Can you work these out from the model? Positions are in its coordinate system, mm. A direction names the side the tool comes from. Give positions to 0.01 mm unless a question says otherwise; leave off trailing zeros. Order: outer loops, then holes, each group sorted by start corner. A loop starts at its lowest first (then second) coordinate and runs counter-clockwise, first axis right, second up. Notation, with made-up numbers: M -17.75,31.25 L 35.25,31.25 A10 ccw 35.25,49.25 Z; hole C 16.5,10 d9. An arc over 180 degrees is marked long. Answer as a JSON object with one key per item and string values.
```python
from build123d import *

# Parameters (mm, degrees)
SKETCH_1_W          = 10
SKETCH_1_H          = 19
EXTRUDE_1_DEPTH     = 10
SKETCH_3_R          = 2.1
CUT_EXTRUDE_2_DEPTH = 15.671400751
CUT_EXTRUDE_4_DEPTH = 5
SKETCH_2_R          = 1.5
CUT_EXTRUDE_1_DEPTH = 10


with BuildPart() as part:
    # 草图1 → 凸台-拉伸1 (new body)
    with BuildSketch(Plane.XY):
        Rectangle(SKETCH_1_W, SKETCH_1_H)
    extrude(amount=EXTRUDE_1_DEPTH)

    # 草图3 → 切除-拉伸2 (cut, through all)
    with BuildSketch(Plane(origin=(0, 0, 0), x_dir=(-1, 0, 0), z_dir=(0, 0, -1))):
        with Locations((0, 6)):
            Circle(SKETCH_3_R)
    extrude(amount=-CUT_EXTRUDE_2_DEPTH, mode=Mode.SUBTRACT)

    # 草图6 → 切除-拉伸4 (cut)
    with BuildSketch(Plane(origin=(0, 0, 0), x_dir=(-1, 0, 0), z_dir=(0, 0, -1))):
        Polygon((5, 9.5), (-5, 9.5), (-5, -1.5), (-2, 0.5), (2, 0.5), (5, -1.5), align=None)
    extrude(amount=-CUT_EXTRUDE_4_DEPTH, mode=Mode.SUBTRACT)

    # 草图2 → 切除-拉伸1 (cut)
    with BuildSketch(Plane.XZ.offset(9.5)):
        with Locations(Location((0, 5, 0), (0, 0, 270))):
            Circle(SKETCH_2_R)
    extrude(amount=-CUT_EXTRUDE_1_DEPTH, mode=Mode.SUBTRACT)


solid = part.part
```
1) I want a section at D-D on x = 1.75. Write out the boundary of the cut face in (y, z), and give its area (3 significant figures).
Results found:
{"outline": "M -9.5,0 L 0.5,0 L 0.5,5 L 4.84,5 L 4.84,10 L -9.5,10 Z; M 7.16,5 L 9.5,5 L 9.5,10 L 7.16,10 Z", "area": "133 mm²"}
2) I need wall thicknesses on L1, parallel to X at y = -5, z = 5; L2, parallel to Y at x = 0, z = 7.75; L3, parallel to Z at x = 1, y = 3.25. Which ranges of each line are inside material? Lowest first, please.
Results found:
{"L1": "x = -5 to -1.5, 1.5 to 5", "L2": "y = -9.5 to 3.9, 8.1 to 9.5", "L3": "z = 5 to 10"}
3) I want a section at C-C on z = 5.75. Write out the boundary of the cut face in (x, y), and give its area (3 significant figures).
Results found:
{"outline": "M -5,-9.5 L -1.3,-9.5 L -1.3,0.5 L 1.3,0.5 L 1.3,-9.5 L 5,-9.5 L 5,9.5 L -5,9.5 Z; hole C 0,6 d4.2", "area": "150 mm²"}
4) Thinking about a two-plate mould opening in X: for faces 1 (the face through (-3.5, -0.5, 2.5)), 2 (the face through (5, -2, 6)), 3 (the face through (0, 0.5, 6)), 4 (the face through (0.07, -4.57, 6.5)), which applies, pulls with the +X half, pulls with the -X half, needs draft (parallel to the pull), parting line crosses it, or undercut?
Results found:
{"face 1": "pulls with the -X half", "face 2": "pulls with the +X half", "face 3": "undercut", "face 4": "undercut"}
5) I want a section at B-B on x = 0. Write out the boundary of the cut face in (y, z), and give its area (3 significant figures).
Results found:
{"outline": "M -9.5,0 L 0.5,0 L 0.5,3.5 L -9.5,3.5 Z; M -9.5,6.5 L 0.5,6.5 L 0.5,5 L 3.9,5 L 3.9,10 L -9.5,10 Z; M 8.1,5 L 9.5,5 L 9.5,10 L 8.1,10 Z", "area": "94.0 mm²"}
6) I'm going to push flat-ended pins straight in: pin 1 Ø1.2 at (x, z) = (1, 3) entering from +Y; pin 2 Ø2 at (y, z) = (2.5, 2) entering from -X. Where does each tip first touch, or does it pass through?
Results found:
{"pin 1": "stops at y = 0.5", "pin 2": "passes through"}
7) I want a section at A-A on y = 6. Write out the boundary of the cut face in (x, z).
Results found:
{"outline": "M -5,5 L -2.1,5 L -2.1,10 L -5,10 Z; M 2.1,5 L 5,5 L 5,10 L 2.1,10 Z"}
8) For faces 5 (the face through (0, 0.5, 2)), 6 (the face through (-1.2, -9.5, 3.8)), 7 (the face through (3.5, -0.5, 2.5)), which set-ups out of +Z, -Z, +X, -X, +Y, -Y let a thin tool reach every point of the face, with its end or its side?
Results found:
{"face 5": "-Z, +X, -X, +Y", "face 6": "+Z, -Z, +X, -X, -Y", "face 7": "-Z, +X, +Y"}
